Input: part model. Units: mm. Frame: model coordinates. A direction names the side the tool comes from. Give positions to 0.01 mm unless a question says otherwise; leave off trailing zeros. Write each loop counter-clockwise with the first axis right and the second up, starting at its lowest first coordinate (ties: lowest second). Pieces come first, ordered by that corner, then holes.
```python
from build123d import *

# Parameters (mm, degrees)
SKETCH1_R           = 1.205
BOSS_EXTRUDE1_DEPTH = 2
SKETCH2_W           = 4.74
SKETCH2_H           = 5
SKETCH2_R           = 0.271758231
BOSS_EXTRUDE2_DEPTH = 4


with BuildPart() as part:
    # Sketch1 → Boss-Extrude1 (new body)
    with BuildSketch(Plane(origin=(0, 0, 0), x_dir=(1, 0, 0), z_dir=(0, 1, 0))):
        with BuildLine():
            Line((-11.85, 14), (11.85, 14))
            ThreePointArc((11.85, 14), (12.557106781, 13.707106781), (12.85, 13))
            Line((12.85, 13), (12.85, -13))
            ThreePointArc((12.85, -13), (12.557106781, -13.707106781), (11.85, -14))
            Line((11.85, -14), (-11.85, -14))
            ThreePointArc((-11.85, -14), (-12.557106781, -13.707106781), (-12.85, -13))
            Line((-12.85, -13), (-12.85, 13))
            ThreePointArc((-12.85, 13), (-12.557106781, 13.707106781), (-11.85, 14))
        make_face()
        with Locations((-10.105, 11.46)):
            Circle(SKETCH1_R, mode=Mode.SUBTRACT)
        with Locations((-10.105, -11.46)):
            Circle(SKETCH1_R, mode=Mode.SUBTRACT)
        with Locations((10.026555832, -11.46)):
            Circle(SKETCH1_R, mode=Mode.SUBTRACT)
        with Locations((10.105, 11.46)):
            Circle(SKETCH1_R, mode=Mode.SUBTRACT)
    extrude(amount=BOSS_EXTRUDE1_DEPTH)

    # Sketch2 → Boss-Extrude2 (add)
    with BuildSketch(Plane(origin=(0, 0, 0), x_dir=(1, 0, 0), z_dir=(0, 1, 0))):
        Rectangle(SKETCH2_W, SKETCH2_H)
        with Locations((-0.548413106, 0)):
            Circle(SKETCH2_R, mode=Mode.SUBTRACT)
    extrude(amount=BOSS_EXTRUDE2_DEPTH)


solid = part.part
```
Q1. Section B-B, the plane y = 0.8. Return the cut outline in (x, z) (3 decimals).
Q2. Mould query, pull axis Z, two halves, no side actions, for faces 1 (the flat face through (0, 3, 2.5)), 2 (the flat face through (-3, 2, 0)), 3 (the cylindrical face through (-8.956, 0.986, 11.098)). Classes: +Z half, -Z half, draft (parallel to the pull), parting line (faces both ways), or undercut.
Q3. Material intervals for line 1 along X through (y, z) = (0.7, -11.46); line 2 along X through (y, z) = (1.05, 11.46); line 3 along X through (y, z) = (2.95, 0), sorted ascending.
Q4. Pin query (flat end, axial travel): pin 1 (1.6 mm diameter, centred on y = 3, z = 0, fed in from +X); pin 2 (10 mm diameter, centred on x = -5, z = -7, fed in from +Y); pin 3 (1 mm diameter, centred on x = -0.5, y = 3, fed in from -Z). Return the tip coordinate at first contact, or that it passes through.
Q5. Section D-D, the plane x = -4.5. Return the cut outline in (y, z).
Q6. Section C-C, the plane x = 2. Return the cut outline in (y, z).
Q7. Access query for faces 4 (the flat face through (-2.37, 3, 0)), 5 (the flat face through (2.37, 3, 0)), 6 (the flat face through (0, 3, -2.5)), 7 (the cylindrical face through (12.565, 0.986, 13.699)). Directions: +Z, -Z, +X, -X, +Y, -Y. A direction counts if a zero-diameter tool reaches every point of the face in a straight line with its end or side. Return the directions, or none.
Q8. Section A-A, the plane z = 11.46. Return the cut outline in (x, y), then the cut area to 3 significant figures.
Solutions:
1. outline: (-12.85, -13) arc R1 ccw to (-11.85, -14) - (11.85, -14) arc R1 ccw to (12.85, -13) - (12.85, 13) arc R1 ccw to (11.85, 14) - (-11.85, 14) arc R1 ccw to (-12.85, 13) - close; hole circle Ø2.41 at (-10.105, -11.46); hole circle Ø2.41 at (-10.105, 11.46); hole circle Ø2.41 at (10.027, 11.46); hole circle Ø2.41 at (10.105, -11.46)
2. face 1: +Z half
2. face 2: draft
2. face 3: undercut
3. line 1: x = -12.85 to -11.31, -8.9 to 8.9, 11.31 to 12.85
3. line 2: x = -12.85 to -11.31, -8.9 to 8.82, 11.23 to 12.85
3. line 3: x = -2.37 to -0.82, -0.28 to 2.37
4. pin 1: stops at x = 2.37
4. pin 2: stops at y = 2
4. pin 3: stops at z = -2.5
5. outline: (0, -14) - (2, -14) - (2, 14) - (0, 14) - close
6. outline: (0, -14) - (2, -14) - (2, -2.5) - (4, -2.5) - (4, 2.5) - (2, 2.5) - (2, 14) - (0, 14) - close
7. face 4: +Z, -Z, -X, +Y
7. face 5: +Z, -Z, +X, +Y
7. face 6: -Z, +X, -X, +Y
7. face 7: +Z, +X, +Y, -Y
8. outline: (-12.85, 0) - (-11.31, 0) - (-11.31, 2) - (-12.85, 2) - close; (-8.9, 0) - (8.82, 0) - (8.82, 2) - (-8.9, 2) - close; (11.23, 0) - (12.85, 0) - (12.85, 2) - (11.23, 2) - close
8. area: 41.8 mm2
